```python
from build123d import *

# Parameters (mm, degrees)
BOSS_EXTRUDE1_REACH      = 56.083
BOSS_EXTRUDE1_END_RADIUS = 20
SKETCH2_R                = 10
SKETCH3_R                = 5
BOSS_EXTRUDE2_DEPTH      = 50


with BuildPart() as part:
    # Sketch1 → Revolve1 (revolve)
    with BuildSketch(Plane.XY):
        with BuildLine():
            Line((-5, 20), (5, 20))
            Line((5, 20), (5, 14.142135624))
            ThreePointArc((5, 14.142135624), (0, 15), (-5, 14.142135624))
            Line((-5, 14.142135624), (-5, 20))
        make_face()
    revolve(axis=Axis((25.861561119, 0, 0), (-1, 0, 0)))

    # Boss-Extrude1: up to this cylinder (the profile starts outside it)
    boss_extrude1_end = Plane(origin=(0, 0, 0), z_dir=(1, 0, 0)) * Cylinder(BOSS_EXTRUDE1_END_RADIUS, 153.166, mode=Mode.PRIVATE)
    # Sketch2 → Boss-Extrude1 (add, up to the surface)
    with BuildSketch(Plane.XY.offset(30), mode=Mode.PRIVATE) as boss_extrude1_sk1:
        Circle(SKETCH2_R)
    boss_extrude1_tool1 = extrude(boss_extrude1_sk1.sketch, amount=-BOSS_EXTRUDE1_REACH, mode=Mode.PRIVATE) - boss_extrude1_end
    add(boss_extrude1_tool1.solids().sort_by_distance((0, 0, 30))[0])

    # Sketch3 → Boss-Extrude2 (add)
    with BuildSketch(Plane.XY.offset(30)):
        Circle(SKETCH3_R)
    extrude(amount=BOSS_EXTRUDE2_DEPTH)


solid = part.part
```
CAD build for the part. Positions are in the model's coordinates, mm. A direction names the side the tool comes from. Round coordinates to 2 decimals unless told otherwise and drop trailing zeros. Write each loop counter-clockwise with the first axis right and the second up, starting at its lowest first coordinate (ties: lowest second). Pieces come first, ordered by that corner, then holes.
Item 1: Band-saw the part on C-C on z = 8.5. Write the cut outline in (x, y), then the cut area to 3 significant figures.
Filled in:
outline: (-5, -18.1) - (5, -18.1) - (5, -11.3) arc R12.36 cw to (-5, -11.3) - close; (-5, 11.3) arc R12.36 cw to (5, 11.3) - (5, 18.1) - (-5, 18.1) - close
area: 122 mm2
Item 2: Mould opens along Y. For faces 1 (the flat face through (0, 0, 80)), 2 (the cylindrical face through (-7, 0, 20)), 3 (the cylindrical face through (-1.08, -4.88, 54.65)) say: released by +Y, released by -Y, zero draft, split by the parting line, or undercut.
Filled in:
face 1: zero draft
face 2: undercut
face 3: split by the parting line
Item 3: Drop flat-ended pins along their axis: pin 1 Ø12 at (x, z) = (6.5, 19) entering from +Y; pin 2 Ø2 at (x, z) = (5, 66.5) entering from +Y; pin 3 Ø12 at (x, z) = (-4, 34) entering from -Y; pin 4 Ø12 at (y, z) = (-2, -2) entering from +X. Give the stop position or say it passes through.
Filled in:
pin 1: stops at y = 15.03
pin 2: stops at y = 3
pin 3: stops at y = -10
pin 4: passes through
Item 4: Tool access for faces 4 (the flat face through (-5, -2, 30)), 5 (the cylindrical face through (7, 0, 20)): list every direction of +Z, -Z, +X, -X, +Y, -Y with a clear straight run to the whole face (end or side of a thin tool).
Filled in:
face 4: +Z
face 5: -Z, +X
Item 5: Band-saw the part on B-B on y = 6. Write the cut outline in (x, z).
Filled in:
outline: (-8, 19.08) - (-5, 19.08) - (-5, 12.81) arc R13.75 cw to (5, 12.81) - (5, 19.08) - (8, 19.08) - (8, 30) - (-8, 30) - close; (-5, -19.08) - (5, -19.08) - (5, -12.81) arc R13.75 cw to (-5, -12.81) - close
Item 6: Band-saw the part on A-A on x = 0. Write the cut outline in (y, z).
Filled in:
outline: (-10, 17.32) arc R20 ccw (long way) to (10, 17.32) - (10, 30) - (5, 30) - (5, 80) - (-5, 80) - (-5, 30) - (-10, 30) - close; hole circle Ø30 at (0, 0)
Item 7: Band-saw the part on D-D on z = 52. Write the cut outline in (x, y), then the cut area to 3 significant figures.
Filled in:
outline: circle Ø10 at (0, 0)
area: 78.5 mm2
Item 8: Drill centre lines: L1, parallel to X at y = -13, z = -11; L2, parallel to Z at x = -1.25, y = 5; L3, parallel to Y at x = 3.25, z = 4. Where is each one in solid material? Low to high.
Filled in:
L1: x = -5 to 5
L2: z = -19.36 to -14.09, 14.09 to 30
L3: y = -19.6 to -14.09, 14.09 to 19.6
